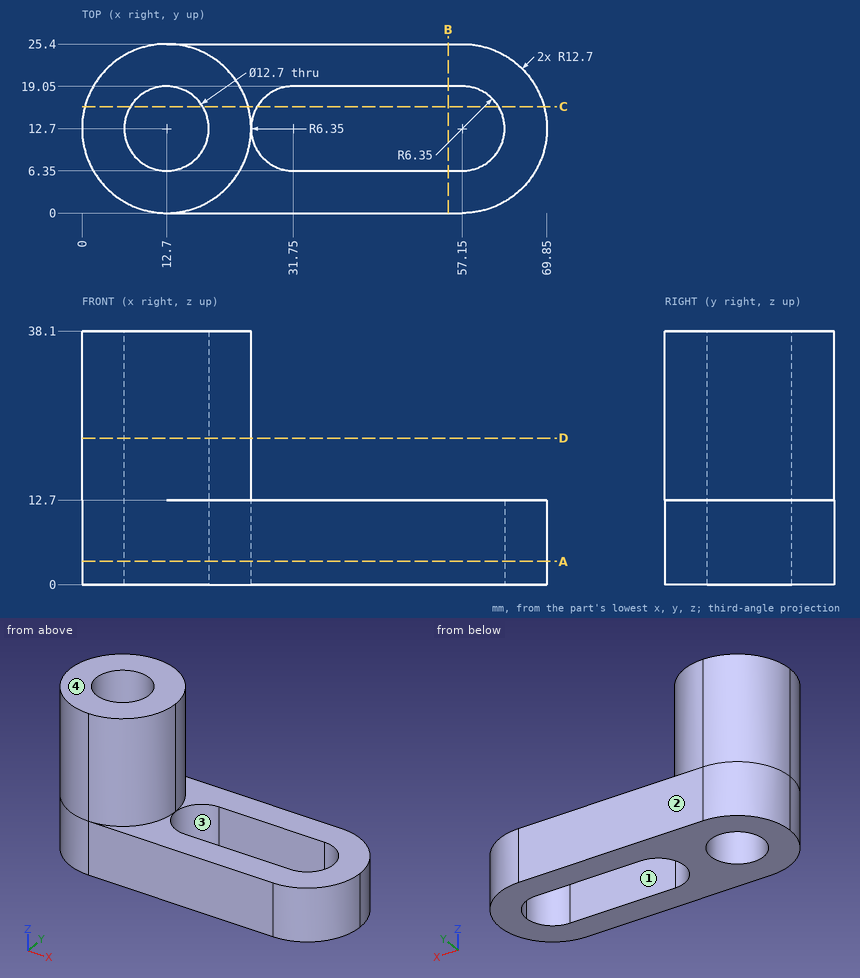
Could you check a few things on this drawing? It's one solid part, dimensions in mm from its lowest x, y, z. A direction names the side the tool comes from. Round coordinates to 2 decimals unless told otherwise and drop trailing zeros. Write each loop counter-clockwise with the first axis right and the second up, starting at its lowest first coordinate (ties: lowest second). Pieces come first, ordered by that corner, then holes. Notation, with made-up numbers: M -15,-31 L 5,-31 A12 cw 5,-9 Z; hole C 29,89.25 d3. An arc over 180 degrees is marked long. Answer as CSV lines item,"result". Start each with the question number.
1. Suppose I cut it at C-C on y = 16. Write out the boundary of the cut face in (x, z).
2. I need wall thicknesses on probe 1 along Z at (x, y) = (30.5, 5); probe 2 along Y at (x, z) = (47, 2); probe 3 along Y at (x, z) = (31, 3). Which ranges of each line are inside material? Lowest first, please.
3. Suppose I cut it at A-A on z = 3.5. Write out the boundary of the cut face in (x, y), then the cut area to 3 significant figures.
4. I'm going to push flat-ended pins straight in: pin 1 Ø8 at (y, z) = (8.5, 7) entering from +X; pin 2 Ø1 at (y, z) = (19, 23.5) entering from +X; pin 3 Ø1.5 at (y, z) = (22, 19.5) entering from +X. Where does each tip first touch, or does it pass through?
5. Thinking about a two-plate mould opening in X: for the marked faces 1 and 2, which applies, released by +X, released by -X, zero draft, split by the parting line, or undercut?
6. Suppose I cut it at D-D on z = 22. Write out the boundary of the cut face in (x, y).
7. On a 3-axis mill with a long thin cutter (end or side, diameter ignored), from which of +Z, -Z, +X, -X, +Y, -Y can I reach the whole of each face in a straight line? I mean the marked faces 3 and 4. Say none if no direction works.
8. Suppose I cut it at B-B on x = 55. Write out the boundary of the cut face in (y, z), then the cut area to 3 significant figures.
Check result:
1,outline,"M 0.44,0 L 7.27,0 L 7.27,38.1 L 0.44,38.1 Z; M 18.13,0 L 26.32,0 L 26.32,12.7 L 24.96,12.7 L 24.96,38.1 L 18.13,38.1 Z; M 62.58,0 L 69.41,0 L 69.41,12.7 L 62.58,12.7 Z"
2,probe 1,"z = 0 to 12.7"
2,probe 2,"y = 0 to 6.35, 19.05 to 25.4"
2,probe 3,"y = 0 to 6.39, 19.01 to 25.4"
3,outline,"M 12.7,0 L 57.15,0 A12.7 ccw 57.15,25.4 L 12.7,25.4 A12.7 ccw Z; hole C 12.7,12.7 d12.7; hole M 31.75,6.35 L 57.15,6.35 A6.35 ccw 57.15,19.05 L 31.75,19.05 A6.35 ccw Z"
3,area,"1,060 mm2"
4,pin 1,"stops at x = 69.85"
4,pin 2,"stops at x = 24"
4,pin 3,"stops at x = 22.09"
5,face 1,"undercut"
5,face 2,"zero draft"
6,outline,"C 12.7,12.7 d25.4; hole C 12.7,12.7 d12.7"
7,face 3,"+Z, -Z"
7,face 4,"+Z, +X, -X, +Y, -Y"
8,outline,"M 0,0 L 6.35,0 L 6.35,12.7 L 0,12.7 Z; M 19.05,0 L 25.4,0 L 25.4,12.7 L 19.05,12.7 Z"
8,area,"161 mm2"
